CAD build for the part. Positions are in the model's coordinates, mm. A direction names the side the tool comes from. Round coordinates to 2 decimals unless told otherwise and drop trailing zeros. Order: outer loops, then holes, each group sorted by start corner. A loop starts at its lowest first (then second) coordinate and runs counter-clockwise, first axis right, second up. Notation, with made-up numbers: M 59.5,83.25 L 94.5,83.25 A35 ccw 94.5,117.25 Z; hole C -31.5,-36.5 d1. An arc over 180 degrees is marked long. Answer as a JSON object with one key per item and string values. Group by question number.
```python
from build123d import *

# Parameters (mm, degrees)
F0_W     = 104.775
F0_H     = 76.2
F1_DEPTH = 25.4
F2_W     = 25.4
F2_H     = 76.2
F3_DEPTH = 4.7752
F5_D     = 6.5278


with BuildPart() as f1:
    # F0 (on Front) → F1 (new body)
    with BuildSketch(Plane.XZ):
        Rectangle(F0_W, F0_H)
    extrude(amount=F1_DEPTH)

    # F2 (on face) → F3 (cut)
    with BuildSketch(Plane.XZ.offset(25.4)):
        with Locations((39.6875, 0)):
            Rectangle(F2_W, F2_H)
    extrude(amount=-F3_DEPTH, mode=Mode.SUBTRACT)

    # F5 (through all)
    with Locations(Plane.XZ.offset(20.6248)):
        with Locations((45.2501, -12.954), (45.2501, 12.954)):
            Hole(F5_D / 2)


solid = f1.part
```
Item 1: Cut at B-B, the plane z = -32.5. Give the cut face in (x, y), and give its area (3 significant figures).
Item 2: Cut at C-C, the plane x = 37. Give the cut face in (y, z).
Item 3: Drill centre lines: line 1 (Z direction, x = 46, y = -5); line 2 (Z direction, x = 46.5, y = -15.5); line 3 (X direction, y = -22.5, z = 1.5). Where is each one in solid material? Low to high. Write a range as [from, to].
Item 4: 3-axis set-ups, long thin cutter, end or side, ignore diameter. For faces 1 (the face through (48.51, -10.17, -12.81)), 2 (the face through (40, -20.625, 1)): which of +Z, -Z, +X, -X, +Y, -Y reach the whole face in a straight line?
Item 5: Flat gauge pins, fed straight in: pin 1 Ø10 at (y, z) = (-22, 2.5) entering from +X; pin 2 Ø1.4 at (y, z) = (-22, 18) entering from +X. Where does each tip first touch, or does it go through?
Item 6: Cut at A-A, the plane z = 11. Give the cut face in (x, y).
Item 7: Cut at D-D, the plane y = -22.75. Give the cut face in (x, z), and give its area (3 significant figures).
Item 8: Two-plate mould, pull along X, no slides. Class faces 3 (the face through (-1, -13, -38.1)), 4 (the face through (26.988, -23, -1)), 5 (the face through (48.51, -10.17, 13.1)): +X half, -X half, draft (parallel to the pull), parting line (faces both ways), or undercut.
Response values:
{
 "1": {"outline": "M -52.39,-25.4 L 26.99,-25.4 L 26.99,-20.62 L 52.39,-20.62 L 52.39,0 L -52.39,0 Z", "area": "2,540 mm^2"},
 "2": {"outline": "M -20.62,-38.1 L 0,-38.1 L 0,38.1 L -20.62,38.1 Z"},
 "3": {"line 1": "[-38.1, -16.13], [-9.78, 9.78], [16.13, 38.1]", "line 2": "[-38.1, -15.97], [-9.94, 9.94], [15.97, 38.1]", "line 3": "[-52.39, 26.99]"},
 "4": {"face 1": "+Y, -Y", "face 2": "+Z, -Z, +X, -Y"},
 "5": {"pin 1": "x = 52.39", "pin 2": "x = 26.99"},
 "6": {"outline": "M -52.39,-25.4 L 26.99,-25.4 L 26.99,-20.62 L 42.64,-20.62 L 42.64,0 L -52.39,0 Z; M 47.86,-20.62 L 52.39,-20.62 L 52.39,0 L 47.86,0 Z"},
 "7": {"outline": "M -52.39,-38.1 L 26.99,-38.1 L 26.99,38.1 L -52.39,38.1 Z", "area": "6,050 mm^2"},
 "8": {"face 3": "draft", "face 4": "+X half", "face 5": "undercut"}
}
